CAD build for the part. Positions are in the model's coordinates, mm. A direction names the side the tool comes from. Give positions to 0.01 mm unless a question says otherwise; leave off trailing zeros. Order: outer loops, then holes, each group sorted by start corner. A loop starts at its lowest first (then second) coordinate and runs counter-clockwise, first axis right, second up.
from build123d import *

# Parameters (mm, degrees)
BOSS_EXTRU_1_DEPTH      = 80
ENL_V_MAT_EXTRU_1_DEPTH = 9
D_GAGEMENT_M41_D        = 4.5
D_GAGEMENT_M41_DEPTH    = 10
D_GAGEMENT_M41_TIP      = 1.351936393
ENL_V_MAT_EXTRU_2_DEPTH = 4
D_GAGEMENT_M42_D        = 4.4
D_GAGEMENT_M42_DEPTH    = 10
D_GAGEMENT_M42_TIP      = 1.321893362


with BuildPart() as part:
    # Esquisse1 → Boss.-Extru.1 (new body)
    with BuildSketch(Plane(origin=(0, 0, 0), x_dir=(0, 0, -1), z_dir=(1, 0, 0))):
        Polygon((-33.838993879, -37.26557224), (-14.838993879, -37.26557224), (-14.838993879, -17.26557224), (-21.838993879, -17.26557224), (-21.838993879, -20.26557224), (-27.838993879, -20.26557224), (-27.838993879, -17.26557224), (-34.838993879, -17.26557224), (-34.838993879, 11.73442776), (-26.838993879, 11.73442776), (-26.838993879, -8.26557224), (-21.838993879, -13.26557224), (-10.838993879, -13.26557224), (-10.838993879, -41.26557224), (-33.838993879, -41.26557224), align=None)
    extrude(amount=BOSS_EXTRU_1_DEPTH)

    # Esquisse2 → Enlèv. mat.-Extru.1 (cut, through all)
    with BuildSketch(Plane(origin=(0, 0, 26.838993879), x_dir=(-1, 0, 0), z_dir=(0, 0, -1))):
        Polygon((-80, -8.26557224), (-44, 11.73442776), (-36, 11.73442776), (0, -8.26557224), (0, 11.73442776), (-36, 16.436885369), (-44, 16.436885369), (-80, 11.73442776), align=None)
    extrude(amount=-ENL_V_MAT_EXTRU_1_DEPTH, mode=Mode.SUBTRACT)

    # Dégagement M41
    with Locations(Plane(origin=(0, 0, 26.838993879), x_dir=(-1, 0, 0), z_dir=(0, 0, -1))):
        with Locations((-40, 2.73442776)):
            Hole(D_GAGEMENT_M41_D / 2, depth=D_GAGEMENT_M41_DEPTH)
            with Locations((0, 0, -(D_GAGEMENT_M41_DEPTH + D_GAGEMENT_M41_TIP / 2))):  # 118° drill point
                Cone(0, D_GAGEMENT_M41_D / 2, D_GAGEMENT_M41_TIP, mode=Mode.SUBTRACT)

    # Esquisse7 → Enlèv. mat.-Extru.2 (cut)
    with BuildSketch(Plane(origin=(0, 0, 26.838993879), x_dir=(-1, 0, 0), z_dir=(0, 0, -1))):
        Polygon((-40, 6.73442776), (-43.464101615, 4.73442776), (-43.464101615, 0.73442776), (-40, -1.26557224), (-36.535898385, 0.73442776), (-36.535898385, 4.73442776), align=None)
    extrude(amount=-ENL_V_MAT_EXTRU_2_DEPTH, mode=Mode.SUBTRACT)

    # Dégagement M42
    with Locations(Plane(origin=(0, -41.26557224, 0), x_dir=(-1, 0, 0), z_dir=(0, -1, 0))):
        with Locations((-10, -24.838993879), (-40, -24.838993879), (-70, -24.838993879)):
            Hole(D_GAGEMENT_M42_D / 2, depth=D_GAGEMENT_M42_DEPTH)
            with Locations((0, 0, -(D_GAGEMENT_M42_DEPTH + D_GAGEMENT_M42_TIP / 2))):  # 118° drill point
                Cone(0, D_GAGEMENT_M42_D / 2, D_GAGEMENT_M42_TIP, mode=Mode.SUBTRACT)


solid = part.part
1. Saw through at C-C on y = -26. Give the cut face in (x, z).
2. 3-axis set-ups, long thin cutter, end or side, ignore diameter. For faces 4 (the flat face through (36.536, 3, 29)), 5 (the flat face through (39, -19, 21.839)), 6 (the flat face through (39, -37.266, 22)), 7 (the flat face through (39, -3, 26.839)), 8 (the cylindrical face through (37.802, -39.238, 24.742)): which of +Z, -Z, +X, -X, +Y, -Y reach the whole face in a straight line?
3. Pin check, flat tips, straight feed: P1, Ø3.5, axis at x = 41, y = 3.5, coming from the -Z side; P2, Ø7, axis at x = 40, y = 2.73, coming from the -Z side; P3, Ø5, axis at x = 9, z = 17, coming from the +Y side. Stop position of each tip, or through.
4. Saw through at D-D on x = 19. Give the cut face in (y, z).
5. Wall check: line 1 (Y direction, x = 40, z = 32.4); line 2 (Y direction, x = 44, z = 33.5); line 3 (Z direction, x = 70, y = -39). Give the ranges that are in metal, low to high.
6. Mould opens along Y. For faces 1 (the cylindrical face through (7.802, -39.238, 24.742)), 2 (the flat face through (42, 1, 30.839)), 3 (the flat face through (40, 11.734, 31)) say: released by +Y, released by -Y, zero draft, split by the parting line, or undercut.
7. Saw through at A-A on z = 32.5. Give the cut face in (x, y), plus the area to 3 significant figures.
8. Saw through at B-B on x = 65. Give the cut face in (y, z), plus the area to 3 significant figures.
Reported:
1. outline: (0, 10.84) - (80, 10.84) - (80, 14.84) - (0, 14.84) - close
2. face 4: -Z
2. face 5: +X, -X
2. face 6: +Z, +X, -X
2. face 7: -Z, +X, -X, +Y
2. face 8: -Y
3. P1: stops at z = 30.84
3. P2: stops at z = 26.84
3. P3: stops at y = -13.27
4. outline: (-41.27, 10.84) - (-13.27, 10.84) - (-13.27, 21.84) - (-8.27, 26.84) - (2.29, 26.84) - (2.29, 34.84) - (-17.27, 34.84) - (-17.27, 27.84) - (-20.27, 27.84) - (-20.27, 21.84) - (-17.27, 21.84) - (-17.27, 14.84) - (-37.27, 14.84) - (-37.27, 33.84) - (-41.27, 33.84) - close
5. line 1: y = -41.27 to -37.27, -17.27 to 0.48, 4.98 to 11.73
5. line 2: y = -41.27 to -37.27, -17.27 to 11.73
5. line 3: z = 10.84 to 22.64, 27.04 to 33.84
6. face 1: zero draft
6. face 2: undercut
6. face 3: released by +Y
7. outline: (0, -41.27) - (80, -41.27) - (80, -37.27) - (0, -37.27) - close; (0, -17.27) - (80, -17.27) - (80, -8.27) - (44, 11.73) - (36, 11.73) - (0, -8.27) - close; hole circle Ø4.5 at (40, 2.73)
7. area: 1,900 mm2
8. outline: (-41.27, 10.84) - (-13.27, 10.84) - (-13.27, 21.84) - (-8.27, 26.84) - (0.07, 26.84) - (0.07, 34.84) - (-17.27, 34.84) - (-17.27, 27.84) - (-20.27, 27.84) - (-20.27, 21.84) - (-17.27, 21.84) - (-17.27, 14.84) - (-37.27, 14.84) - (-37.27, 33.84) - (-41.27, 33.84) - close
8. area: 405 mm2
